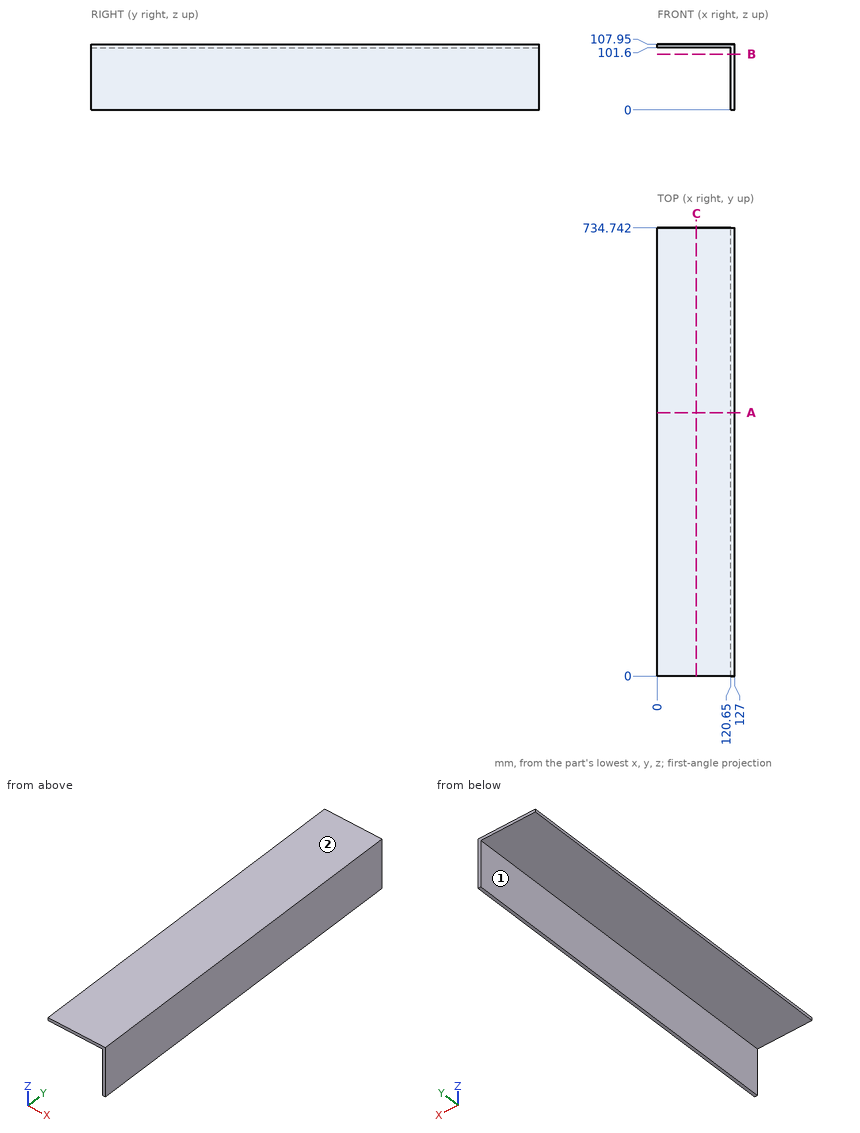
The figure shows three views and two pictorial views of one solid part (mm, origin at its lowest corner). Answer the questions. A direction names the side the tool comes from. Round coordinates to 2 decimals unless told otherwise and drop trailing zeros. Write each loop counter-clockwise with the first axis right and the second up, starting at its lowest first coordinate (ties: lowest second). Pieces come first, ordered by that corner, then holes. Notation, with made-up numbers: M 35,62.5 L 43,62.5 A20 ccw 43,88.5 Z; hole C 47.5,86 d1. An arc over 180 degrees is marked long. Write each question's results on one line, items separated by ' | '. Start each with the question number.
(1) The part is cut by section B-B, the plane z = 91.5. Write down the section's boundary in (x, y), and give its area (3 significant figures).
(2) This flat-tipped pin is pushed along its axis until it touches: P1, Ø4, axis at x = 53, y = 643.5, coming from the -Z side. Where does it stop, or does it pass through?
(3) The part is cut by section C-C, the plane x = 64. Write down the section's boundary in (y, z).
(4) The part is cut by section A-A, the plane y = 432. Write down the section's boundary in (x, z), and give its area (3 significant figures).
(5) For the marked faces 1 and 2, determine the directions among +Z, -Z, +X, -X, +Y, -Y from which every point of the face is accessible in a straight line to the end or side of a thin tool.
(6) Find the intervals of material crossed by line 1 (X direction, y = 680, z = 22); line 2 (Z direction, x = 89.5, y = 697), in increasing order.
Worked answers:
1) outline: M 120.65,0 L 127,0 L 127,734.74 L 120.65,734.74 Z | area: 4,670 mm²
2) P1: stops at z = 101.6
3) outline: M 0,101.6 L 734.74,101.6 L 734.74,107.95 L 0,107.95 Z
4) outline: M 0,101.6 L 120.65,101.6 L 120.65,0 L 127,0 L 127,107.95 L 0,107.95 Z | area: 1,450 mm²
5) face 1: -Z, -X, +Y, -Y | face 2: +Z, +X, -X, +Y, -Y
6) line 1: x = 120.65 to 127 | line 2: z = 101.6 to 107.95
